```python
from build123d import *

# Parameters (mm, degrees)
SKETCH1_W           = 9.525
SKETCH1_H           = 11.0998
BOSS_EXTRUDE1_DEPTH = 0.9398
SKETCH2_W           = 9.525
SKETCH2_H           = 0.9398
BOSS_EXTRUDE2_DEPTH = 17.6784
CUT_EXTRUDE1_DEPTH  = 24.250561203
CUT_EXTRUDE2_DEPTH  = 23.944651046
BOSS_EXTRUDE3_START = 0.9398
SKETCH7_R           = 2.78765
SKETCH7_R_2         = 2.0828
BOSS_EXTRUDE3_DEPTH = 0.9398


with BuildPart() as part:
    # Sketch1 → Boss-Extrude1 (new body)
    with BuildSketch(Plane(origin=(0, 0, 0), x_dir=(1, 0, 0), z_dir=(0, 1, 0))):
        with Locations((4.7625, 5.5499)):
            Rectangle(SKETCH1_W, SKETCH1_H)
    extrude(amount=BOSS_EXTRUDE1_DEPTH)

    # Sketch2 → Boss-Extrude2 (add)
    with BuildSketch(Plane(origin=(0, 0.9398, 0), x_dir=(1, 0, 0), z_dir=(0, 1, 0))):
        with Locations((4.7625, 10.6299)):
            Rectangle(SKETCH2_W, SKETCH2_H)
    extrude(amount=BOSS_EXTRUDE2_DEPTH)

    # Sketch3 → Cut-Extrude1 (cut, through all)
    with BuildSketch(Plane.XY.offset(-10.16)):
        with BuildLine():
            ThreePointArc((6.4897, 15.0622), (5.983814832, 16.283514832), (4.7625, 16.7894))
            Line((4.7625, 16.7894), (4.7625, 13.335))
            ThreePointArc((4.7625, 13.335), (5.983814832, 13.840885168), (6.4897, 15.0622))
        make_face()
        with BuildLine():
            Line((4.7625, 13.335), (4.7625, 16.7894))
            ThreePointArc((4.7625, 16.7894), (3.0353, 15.0622), (4.7625, 13.335))
        make_face()
        with BuildLine():
            ThreePointArc((6.4897, 7.1374), (5.983814832, 8.358714832), (4.7625, 8.8646))
            Line((4.7625, 8.8646), (4.7625, 5.4102))
            ThreePointArc((4.7625, 5.4102), (5.983814832, 5.916085168), (6.4897, 7.1374))
        make_face()
        with BuildLine():
            Line((4.7625, 5.4102), (4.7625, 8.8646))
            ThreePointArc((4.7625, 8.8646), (3.0353, 7.1374), (4.7625, 5.4102))
        make_face()
    extrude(amount=-CUT_EXTRUDE1_DEPTH, mode=Mode.SUBTRACT)

    # Sketch4 → Cut-Extrude2 (cut, through all)
    with BuildSketch(Plane(origin=(0, 0.9398, 0), x_dir=(1, 0, 0), z_dir=(0, 1, 0))):
        with BuildLine():
            ThreePointArc((6.8453, 5.08), (6.235262004, 6.552762004), (4.7625, 7.1628))
            Line((4.7625, 7.1628), (4.7625, 5.08))
            Line((4.7625, 5.08), (6.8453, 5.08))
        make_face()
        with BuildLine():
            Line((4.7625, 5.08), (4.7625, 7.1628))
            ThreePointArc((4.7625, 7.1628), (3.289737996, 6.552762004), (2.6797, 5.08))
            Line((2.6797, 5.08), (4.7625, 5.08))
        make_face()
        with BuildLine():
            Line((6.8453, 5.08), (4.7625, 5.08))
            Line((4.7625, 5.08), (4.7625, 2.9972))
            ThreePointArc((4.7625, 2.9972), (6.235262004, 3.607237996), (6.8453, 5.08))
        make_face()
        with BuildLine():
            Line((4.7625, 2.9972), (4.7625, 5.08))
            Line((4.7625, 5.08), (2.6797, 5.08))
            ThreePointArc((2.6797, 5.08), (3.289737996, 3.607237996), (4.7625, 2.9972))
        make_face()
    extrude(amount=-CUT_EXTRUDE2_DEPTH, mode=Mode.SUBTRACT)

    # Sketch7 → Boss-Extrude3 (add)
    with BuildSketch(Plane(origin=(0, 0.9398, 0), x_dir=(1, 0, 0), z_dir=(0, 1, 0)).offset(BOSS_EXTRUDE3_START)):
        with Locations(Location((4.7625, 5.08, 0), (0, 0, 90))):
            Circle(SKETCH7_R)
        with Locations(Location((4.7625, 5.08, 0), (0, 0, 270))):
            Circle(SKETCH7_R_2, mode=Mode.SUBTRACT)
    extrude(amount=-BOSS_EXTRUDE3_DEPTH)


solid = part.part
```
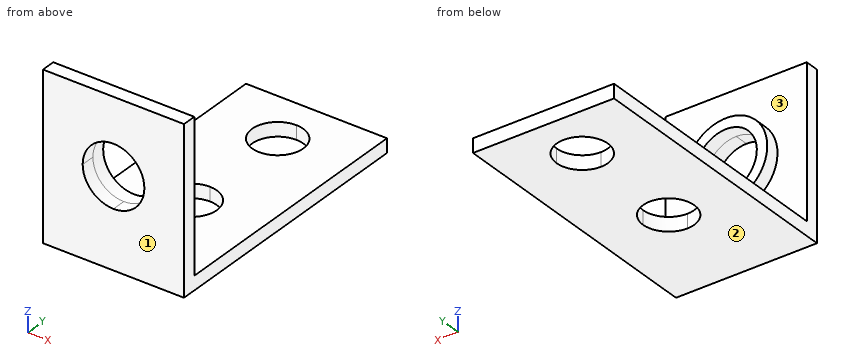
Here's how the part is built. I have some questions about the finished solid (model axes, mm). Face numbers are marked on the shaded views. Round coordinates to 2 decimals unless told otherwise and drop trailing zeros. Write each loop counter-clockwise with the first axis right and the second up, starting at its lowest first coordinate (ties: lowest second). Pieces come first, ordered by that corner, then holes.
Q1. If we section it at D-D on z = -9: Write out the boundary of the cut face in (x, y) (3 decimals), plus the area to 3 significant figures.
Q2. Please list where these lines run through material, in increasing order: probe 1 along X at (y, z) = (1.55, -5.08); probe 2 along Y at (x, z) = (4.5, -10.5); probe 3 along Z at (x, y) = (0.5, 12).
Q3. If we section it at C-C on x = 1.5: Write out the boundary of the cut face in (y, z), plus the area to 3 significant figures.
Q4. Will these pins go through, and if not, where does the flat tip stop? P1, Ø4, axis at x = 7.5, y = 15, coming from the +Z side; P2, Ø3, axis at x = 4, z = -5, coming from the +Y side.
Q5. If we section it at A-A on z = -6: Write out the boundary of the cut face in (x, y) (3 decimals).
Q6. If we mould it in two halves opening along Z, with no side actions, what happens to the marked faces 1, 2 and 3? For each: +Z half, -Z half, draft (parallel to the pull), parting line (faces both ways), or undercut.
Q7. If we section it at B-B on y = 6.75: Write out the boundary of the cut face in (x, z) (3 decimals).
Answer below:
1. outline: (0, 0) - (9.525, 0) - (9.525, 0.94) - (0, 0.94) - close
1. area: 8.95 mm2
2. probe 1: x = 1.97 to 2.68, 6.85 to 7.55
2. probe 2: y = 0 to 5.43, 8.84 to 13.36, 16.77 to 18.62
2. probe 3: z = -11.1 to -10.16
3. outline: (0, -11.1) - (18.62, -11.1) - (18.62, -10.16) - (0.94, -10.16) - (0.94, 0) - (0, 0) - close
3. area: 27.0 mm2
4. P1: stops at z = -10.16
4. P2: stops at y = 1.88
5. outline: (0, 0) - (2.894, 0) - (2.894, 1.88) - (2.131, 1.88) - (2.131, 0.94) - (0, 0.94) - close; (6.631, 0) - (9.525, 0) - (9.525, 0.94) - (7.394, 0.94) - (7.394, 1.88) - (6.631, 1.88) - close
6. face 1: draft
6. face 2: -Z half
6. face 3: undercut
7. outline: (0, -11.1) - (3.079, -11.1) - (3.079, -10.16) - (0, -10.16) - close; (6.446, -11.1) - (9.525, -11.1) - (9.525, -10.16) - (6.446, -10.16) - close
